from build123d import *

# Parameters (mm, degrees)
SKETCH2_R          = 7.9375
CUT_EXTRUDE1_DEPTH = 85.463711951


with BuildPart() as part:
    # Sketch1 → Revolve1 (revolve)
    with BuildSketch(Plane(origin=(0, 0, 0), x_dir=(0, 0, -1), z_dir=(1, 0, 0)), mode=Mode.PRIVATE) as revolve1_sk:
        with BuildLine():
            Line((0, 0), (0, 52.809927725))
            ThreePointArc((0, 52.809927725), (0.130798304, 53.244522907), (0.479738309, 53.534733247))
            Line((0.479738309, 53.534733247), (0.872854821, 53.701601306))
            ThreePointArc((0.872854821, 53.701601306), (1.6002, 54.8005), (0.872854821, 55.899398694))
            Line((0.872854821, 55.899398694), (0.479738309, 56.066266753))
            ThreePointArc((0.479738309, 56.066266753), (0.130798304, 56.356477093), (0, 56.791072275))
            Line((0, 56.791072275), (0, 59.4614))
            Line((0, 59.4614), (2.8448, 59.4614))
            Line((2.8448, 59.4614), (7.9248, 45.504214709))
            Line((7.9248, 45.504214709), (7.9248, 0))
            Line((7.9248, 0), (0, 0))
        make_face()
    revolve(revolve1_sk.sketch.rotate(Axis((0, 0, 0), (0, 0, -1)), 90), axis=Axis((0, 0, 0), (0, 0, -1)))

    # Sketch2 → Cut-Extrude1 (cut, through all)
    with BuildSketch(Plane(origin=(0, 0, -7.9248), x_dir=(-1, 0, 0), z_dir=(0, 0, -1))):
        with Locations((-13.158980507, -27.586296484)):
            Circle(SKETCH2_R)
        with Locations((14.744399845, -27.586296484)):
            Circle(SKETCH2_R)
    extrude(amount=-CUT_EXTRUDE1_DEPTH, mode=Mode.SUBTRACT)


solid = part.part
Could you check a few things on this model? Use its own coordinates, in mm. Coordinates: 2 decimals unless noted, no trailing zeros. Write each loop counter-clockwise with the first axis right and the second up, starting at its lowest first coordinate (ties: lowest second). Pieces come first, ordered by that corner, then holes. Notation, with made-up numbers: (-1.5, 7.25) - (3.5, 7.25) arc R38 cw to (3.5, 45.25) - close; hole circle Ø1 at (4.25, 88). An arc over 180 degrees is marked (long way). Write item = value, one per line.
1) Will these pins go through, and if not, where does the flat tip stop? pin 1 Ø2 at (y, z) = (-24.5, -3.5) entering from -X; pin 2 Ø4 at (y, z) = (-31.5, -3) entering from -X; pin 3 Ø1.5 at (y, z) = (-36, -2) entering from -X.
Result set:
pin_1 = -54.51
pin_2 = -51.62
pin_3 = -47.89
2) Please list where these lines run through material, in increasing order: line 1 (X direction, y = -41, z = -1); line 2 (Y direction, x = -8.5, z = -0.25); line 3 (X direction, y = -49.5, z = -1). Write a range as [from, to].
Result set:
line_1 = [-43.07, -37.9], [-34.78, 34.78], [37.9, 43.07]
line_2 = [-58.85, -55.57], [-52.7, -32.49], [-22.69, 52.7], [55.57, 58.85]
line_3 = [-32.95, -25.83], [-20.99, 20.99], [25.83, 32.95]
3) Suppose I cut it at A-A on y = 0. Please give me the cut outline in (x, z), plus the area to 3 significant figures.
Result set:
outline = (-59.46, -2.84) - (-45.5, -7.92) - (45.5, -7.92) - (59.46, -2.84) - (59.46, 0) - (56.79, 0) arc R0.79 ccw to (56.07, -0.48) - (55.9, -0.87) arc R1.19 cw to (53.7, -0.87) - (53.53, -0.48) arc R0.79 ccw to (52.81, 0) - (-52.81, 0) arc R0.79 ccw to (-53.53, -0.48) - (-53.7, -0.87) arc R1.19 cw to (-55.9, -0.87) - (-56.07, -0.48) arc R0.79 ccw to (-56.79, 0) - (-59.46, 0) - close
area = 865 mm2
4) Suppose I cut it at C-C on y = -21. State how many separate pieces and enclosed holes the cut face has, plus the area to 3 significant figures.
Result set:
separate_pieces = 3
enclosed_holes = 0
area = 657 mm2
5) We'd pull the mould along X, two halves only. Please class faces 1 (the flat face through (-1, -1, -7.925)), 2 (the cylindrical face through (56.716, -17.861, -1.442)), 3 (the cylindrical face through (-8.894, -22.222, -4.018)): +X half, -X half, draft (parallel to the pull), parting line (faces both ways), or undercut.
Result set:
face_1 = draft
face_2 = parting line
face_3 = undercut
